Source: CAD feature listing. Evaluate the final solid. Frame: model axes, mm. Face numbers are marked on the shaded views. Give positions to 0.01 mm unless a question says otherwise; leave off trailing zeros. Write each loop counter-clockwise with the first axis right and the second up, starting at its lowest first coordinate (ties: lowest second). Pieces come first, ordered by that corner, then holes. Notation, with made-up numbers: (71.25, 70) -> (130.25, 70) arc R23 ccw to (130.25, 107) -> close; hole circle Ø6 at (-19, 55). An arc over 180 degrees is marked (long way). Write item = value, one per line.
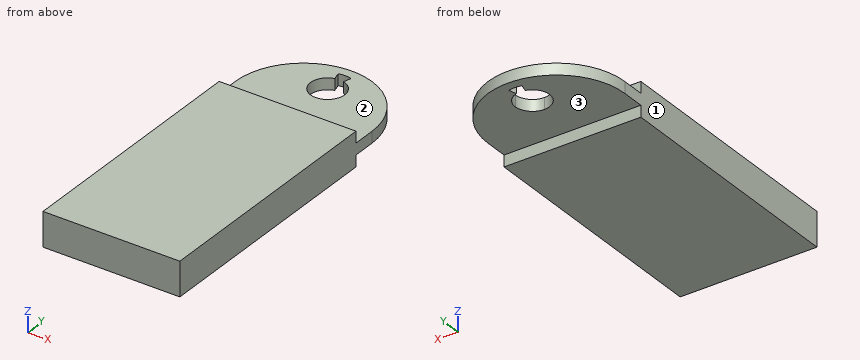
from build123d import *

# Parameters (mm, degrees)
SKETCH_1_W          = 120
SKETCH_1_H          = 240
EXTRUDE_1_DEPTH     = 30
SKETCH_6_W          = 120
SKETCH_6_H          = 10
CUT_EXTRUDE_2_DEPTH = 20
EXTRUDE_4_DEPTH     = 10
CUT_EXTRUDE_3_DEPTH = 327.763219646


with BuildPart() as part:
    # 草图1 → 凸台-拉伸1 (new body)
    with BuildSketch(Plane.XY):
        with Locations((-67.961719718, 120)):
            Rectangle(SKETCH_1_W, SKETCH_1_H)
    extrude(amount=EXTRUDE_1_DEPTH)

    # 草图6 → 切除-拉伸2 (cut)
    with BuildSketch(Plane(origin=(0, 240, 0), x_dir=(1, 0, 0), z_dir=(0, 1, 0))):
        with Locations((-67.961719718, -5)):
            Rectangle(SKETCH_6_W, SKETCH_6_H)
        with Locations((-67.961719718, -25)):
            Rectangle(SKETCH_6_W, SKETCH_6_H)
    extrude(amount=-CUT_EXTRUDE_2_DEPTH, mode=Mode.SUBTRACT)

    # 草图7 → 凸台-拉伸4 (add)
    with BuildSketch(Plane.XY.offset(20)):
        with BuildLine():
            ThreePointArc((-7.961719718, 240), (-67.961719718, 300), (-127.961719718, 240))
            Line((-127.961719718, 240), (-7.961719718, 240))
        make_face()
        with BuildLine():
            Line((-7.961719718, 240), (-127.961719718, 240))
            ThreePointArc((-127.961719718, 240), (-67.961719718, 180), (-7.961719718, 240))
        make_face()
    extrude(amount=-EXTRUDE_4_DEPTH)

    # 草图8 → 切除-拉伸3 (cut, through all)
    with BuildSketch(Plane.XY.offset(20)):
        with BuildLine():
            ThreePointArc((-62.267700726, 291.250368178), (-67.961719718, 292), (-73.65573871, 291.250368178))
            Line((-73.65573871, 291.250368178), (-71.844005395, 284.488887394))
            ThreePointArc((-71.844005395, 284.488887394), (-67.961719718, 285), (-64.079434042, 284.488887394))
            Line((-64.079434042, 284.488887394), (-62.267700726, 291.250368178))
        make_face()
        with BuildLine():
            Line((-71.844005395, 284.488887394), (-67.961719718, 270))
            Line((-67.961719718, 270), (-64.079434042, 284.488887394))
            ThreePointArc((-64.079434042, 284.488887394), (-67.961719718, 285), (-71.844005395, 284.488887394))
        make_face()
        with BuildLine():
            Line((-67.961719718, 270), (-67.961719718, 255))
            ThreePointArc((-67.961719718, 255), (-57.355118, 259.393398282), (-52.961719718, 270))
            ThreePointArc((-52.961719718, 270), (-56.061419614, 279.131421435), (-64.079434042, 284.488887394))
            Line((-64.079434042, 284.488887394), (-67.961719718, 270))
        make_face()
        with BuildLine():
            ThreePointArc((-71.844005395, 284.488887394), (-82.833392639, 268.042107117), (-67.961719718, 255))
            Line((-67.961719718, 255), (-67.961719718, 270))
            Line((-67.961719718, 270), (-71.844005395, 284.488887394))
        make_face()
    extrude(amount=-CUT_EXTRUDE_3_DEPTH, mode=Mode.SUBTRACT)


solid = part.part
1) Cut plane C-C (x = -115). Return the cut outline in (y, z).
Computed:
outline = (0, 0) -> (220, 0) -> (220, 10) -> (277.25, 10) -> (277.25, 20) -> (220, 20) -> (220, 30) -> (0, 30) -> close
2) Material intervals for L1, parallel to Y at x = -41, z = 27.5; L2, parallel to Y at x = -61, z = 11; L3, parallel to Z at x = -55, y = 240, sorted ascending.
Computed:
L1 = 0 to 220
L2 = 0 to 256.71, 283.29 to 299.59
L3 = 10 to 20
3) Cut plane A-A (x = -100). Return the cut outline in (y, z).
Computed:
outline = (0, 0) -> (220, 0) -> (220, 10) -> (290.73, 10) -> (290.73, 20) -> (220, 20) -> (220, 30) -> (0, 30) -> close
4) Cut plane B-B (z = 25.5). Return the cut outline in (x, y).
Computed:
outline = (-127.96, 0) -> (-7.96, 0) -> (-7.96, 220) -> (-127.96, 220) -> close
5) Draft query along Z for the marked faces 1, 2 and 3. Return one class per face: pulls with the +Z half, pulls with the -Z half, needs draft (parallel to the pull), parting line crosses it, or undercut.
Computed:
face_1 = needs draft
face_2 = pulls with the +Z half
face_3 = pulls with the -Z half
6) Contact query for flat-ended pins moving along their axis: pin 1 (3 mm diameter, centred on x = -53.5, z = 7, fed in from +Y); pin 2 (1 mm diameter, centred on y = 259, z = 15, fed in from +X) (3 decimals); pin 3 (24 mm diameter, centred on x = -69, y = 256, fed in from -Z). Output: stop coordinate, or through.
Computed:
pin_1 = 220
pin_2 = -10.885
pin_3 = 10
7) Cut plane D-D (y = 248). Return the cut outline in (x, z).
Computed:
outline = (-127.43, 10) -> (-8.5, 10) -> (-8.5, 20) -> (-127.43, 20) -> close
